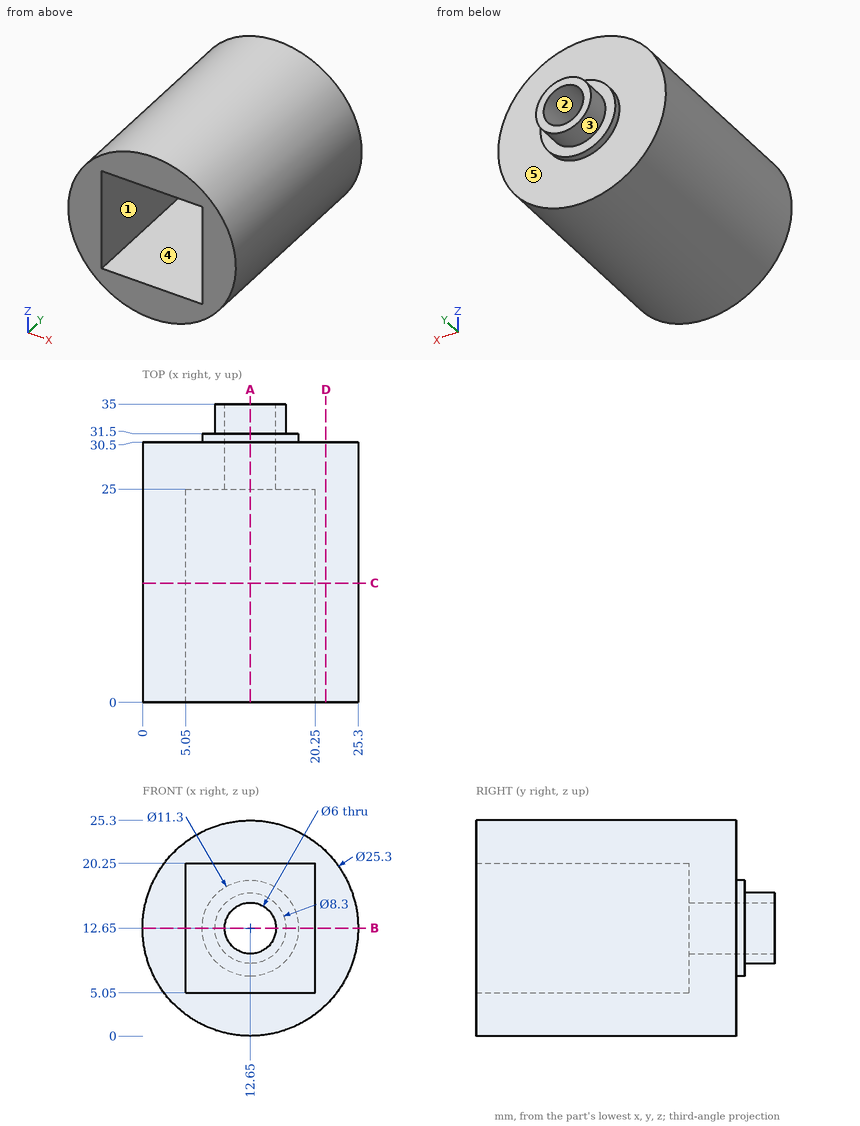
Check sheet for the drawn part. Datum: minimum x, y, z corner. Units: mm. A direction names the side the tool comes from. Round coordinates to 2 decimals unless told otherwise and drop trailing zeros. Loops run counter-clockwise (first coordinate to the right, second up) from the corner with the lowest first, then second, coordinate; pieces in that order, holes last.
Item 1: Cross-section at D-D on x = 21.5. Record the boundary of the cut face in (y, z).
Item 2: Cross-section at A-A on x = 12.65. Record the boundary of the cut face in (y, z).
Item 3: Cross-section at C-C on y = 14. Record the boundary of the cut face in (x, z), then the cut area to 3 significant figures.
Item 4: Gauge pin test, flat ends, axial feed: pin 1 (7.5 mm diameter, centred on y = 11, z = 9, fed in from -X); pin 2 (9.5 mm diameter, centred on x = 12.65, z = 12.65, fed in from -Y); pin 3 (1.5 mm diameter, centred on x = 17.5, z = 4.5, fed in from +Y). Record the tip position at first contact, or that the pin passes through.
Item 5: Mould release check, pull along Z, two halves, no side actions. Record for the marked faces 3, 4 and 5: pulls with the +Z half, pulls with the -Z half, needs draft (parallel to the pull), parting line crosses it, or undercut.
Item 6: Thickness scan on line 1 (X direction, y = 32.25, z = 12.65); line 2 (X direction, y = 28.25, z = 12.65). Record the ranges inside material, lowest first.
Item 7: Access from +Z, -Z, +X, -X, +Y, -Y to the whole of each face (thin tool, end or side, straight path). Record for the marked faces 1 and 2.
Item 8: Cross-section at B-B on z = 12.65. Record the boundary of the cut face in (x, y), then the cut area to 3 significant figures.
Answer sheet:
1. outline: (0, 3.61) - (30.5, 3.61) - (30.5, 21.69) - (0, 21.69) - close
2. outline: (0, 0) - (30.5, 0) - (30.5, 7) - (31.5, 7) - (31.5, 8.5) - (35, 8.5) - (35, 9.65) - (25, 9.65) - (25, 5.05) - (0, 5.05) - close; (0, 20.25) - (25, 20.25) - (25, 15.65) - (35, 15.65) - (35, 16.8) - (31.5, 16.8) - (31.5, 18.3) - (30.5, 18.3) - (30.5, 25.3) - (0, 25.3) - close
3. outline: circle Ø25.3 at (12.65, 12.65); hole (5.05, 5.05) - (20.25, 5.05) - (20.25, 20.25) - (5.05, 20.25) - close
3. area: 272 mm2
4. pin 1: stops at x = 0
4. pin 2: stops at y = 25
4. pin 3: stops at y = 30.5
5. face 3: parting line crosses it
5. face 4: undercut
5. face 5: needs draft
6. line 1: x = 8.5 to 9.65, 15.65 to 16.8
6. line 2: x = 0 to 9.65, 15.65 to 25.3
7. face 1: -Y
7. face 2: +Y, -Y
8. outline: (0, 0) - (5.05, 0) - (5.05, 25) - (9.65, 25) - (9.65, 35) - (8.5, 35) - (8.5, 31.5) - (7, 31.5) - (7, 30.5) - (0, 30.5) - close; (15.65, 25) - (20.25, 25) - (20.25, 0) - (25.3, 0) - (25.3, 30.5) - (18.3, 30.5) - (18.3, 31.5) - (16.8, 31.5) - (16.8, 35) - (15.65, 35) - close
8. area: 372 mm2
